```python
from build123d import *

# Parameters (mm, degrees)
CROQUIS1_W              = 100
CROQUIS1_H              = 100
SALIENTE_EXTRUIR1_DEPTH = 10
CROQUIS2_R              = 5
SALIENTE_EXTRUIR2_DEPTH = 100


with BuildPart() as part:
    # Croquis1 → Saliente-Extruir1 (new body)
    with BuildSketch(Plane(origin=(0, 0, 0), x_dir=(1, 0, 0), z_dir=(0, 1, 0))):
        with Locations((50, 50)):
            Rectangle(CROQUIS1_W, CROQUIS1_H)
    extrude(amount=SALIENTE_EXTRUIR1_DEPTH)

    # Croquis2 → Saliente-Extruir2 (add)
    with BuildSketch(Plane.ZY):
        with Locations(Location((-50, 5, 0), (0, 0, 270))):
            Circle(CROQUIS2_R)
    extrude(amount=SALIENTE_EXTRUIR2_DEPTH)


solid = part.part
```
CAD build for the part. Positions are in the model's coordinates, mm. A direction names the side the tool comes from. Round coordinates to 2 decimals unless told otherwise and drop trailing zeros. Write each loop counter-clockwise with the first axis right and the second up, starting at its lowest first coordinate (ties: lowest second). Pieces come first, ordered by that corner, then holes. Notation, with made-up numbers: (79, -14.5) -> (118, -14.5) arc R22 cw to (118, -4.5) -> close; hole circle Ø5 at (-24, -30.5). An arc over 180 degrees is marked (long way). Answer in a Markdown table with one row per item. Add a question column.
Item 1: Saw through at C-C, the plane z = -12.5. Write the cut outline in (x, y), then the cut area to 3 significant figures.
Item 2: Saw through at B-B, the plane x = -65. Write the cut outline in (y, z), then the cut area to 3 significant figures.
Item 3: Saw through at A-A, the plane y = 5. Write the cut outline in (x, z), then the cut area to 3 significant figures.
Item 4: Drill centre lines: line 1 (X direction, y = 7.5, z = -77); line 2 (Z direction, x = -26, y = 5.5); line 3 (Z direction, x = -5.5, y = 1). Where is each one in solid material? Low to high. Write a range as from..to.
Item 5: Which spindle directions (+Z, -Z, +X, -X, +Y, -Y) get a long thin tool onto all of the face, cutting with end or side? Do faces 1 (the face through (-49.3, 5.651, -45.043)), 2 (the face through (49, 5, 0)). Say none if no direction does.
Item 6: Drop flat-ended pins along their axis: pin 1 Ø5 at (y, z) = (5.5, -79) entering from -X; pin 2 Ø5 at (x, y) = (-44, 3.5) entering from +Z; pin 3 Ø5 at (x, y) = (-68.5, 6) entering from -Z. Give the stop position or say it passes through.
Findings below:
| question | item | result |
|---|---|---|
| 1 | outline | (0, 0) -> (100, 0) -> (100, 10) -> (0, 10) -> close |
| 1 | area | 1,000 mm^2 |
| 2 | outline | circle Ø10 at (5, -50) |
| 2 | area | 78.5 mm^2 |
| 3 | outline | (-100, -55) -> (0, -55) -> (0, -100) -> (100, -100) -> (100, 0) -> (0, 0) -> (0, -45) -> (-100, -45) -> close |
| 3 | area | 11,000 mm^2 |
| 4 | line 1 | x = 0..100 |
| 4 | line 2 | z = -54.97..-45.03 |
| 4 | line 3 | z = -53..-47 |
| 5 | face 1 | -X |
| 5 | face 2 | +Z, +X, -X, +Y, -Y |
| 6 | pin 1 | stops at x = 0 |
| 6 | pin 2 | stops at z = -45 |
| 6 | pin 3 | stops at z = -55 |
